The model under review builds one solid part; all positions refer to its coordinate system, in mm. Face numbers are marked on the shaded views. A direction names the side the tool comes from. Give positions to 0.01 mm unless a question says otherwise; leave off trailing zeros. Order: outer loops, then holes, each group sorted by start corner. A loop starts at its lowest first (then second) coordinate and runs counter-clockwise, first axis right, second up.
```python
from build123d import *

# Parameters (mm, degrees)
BOSS_EXTRUDE1_DEPTH     = 200
BOSS_EXTRUDE2_DEPTH     = 5
BOSS_EXTRUDE3_START     = 200
BOSS_EXTRUDE3_DEPTH     = 5
BOSS_EXTRUDE5_START     = -70
SKETCH12_W              = 5
SKETCH12_H              = 200
BOSS_EXTRUDE5_DEPTH     = 14
SKETCH13_R              = 1.75
SKETCH13_R_2            = 5
SKETCH13_W              = 98
SKETCH13_H              = 41
CUT_EXTRUDE7_DEPTH      = 1
CUT_EXTRUDE7_DEPTH_BACK = 85
SKETCH15_R              = 3
CUT_EXTRUDE8_DEPTH      = 3
SKETCH16_R              = 1.75
CUT_EXTRUDE9_DEPTH      = 111
CUT_EXTRUDE9_DEPTH_BACK = 111
CUT_EXTRUDE10_START     = -103
CUT_EXTRUDE10_DEPTH     = 3
CUT_EXTRUDE11_START     = 100
CUT_EXTRUDE11_DEPTH     = 3
SKETCH18_R              = 3
CUT_EXTRUDE12_DEPTH     = 3


with BuildPart() as part:
    # Sketch1 → Boss-Extrude1 (new body)
    with BuildSketch(Plane(origin=(0, 0, 0), x_dir=(1, 0, 0), z_dir=(0, 1, 0))):
        Polygon((0, 0), (100, 0), (110, 10), (110, 70), (100, 70), (100, 10), (0, 10), align=None)
    boss_extrude1 = extrude(amount=BOSS_EXTRUDE1_DEPTH)

    # Mirror1: Boss-Extrude1 across plane
    add(boss_extrude1.mirror(Plane(origin=(0, 0, 0), x_dir=(0, 0, 1), z_dir=(1, 0, 0))))

    # Sketch6 → Boss-Extrude2 (add)
    with BuildSketch(Plane(origin=(0, 0, 0), x_dir=(1, 0, 0), z_dir=(0, 1, 0))):
        Polygon((110, 70), (-110, 70), (-110, 10), (-100, 0), (100, 0), (110, 10), align=None)
    extrude(amount=-BOSS_EXTRUDE2_DEPTH)

    # Sketch6<2> → Boss-Extrude3 (add)
    with BuildSketch(Plane(origin=(0, 0, 0), x_dir=(1, 0, 0), z_dir=(0, 1, 0)).offset(BOSS_EXTRUDE3_START)):
        Polygon((110, 70), (-110, 70), (-110, 10), (-100, 0), (100, 0), (110, 10), align=None)
    extrude(amount=BOSS_EXTRUDE3_DEPTH)

    # Sketch12 → Boss-Extrude5 (add)
    with BuildSketch(Plane.XY.offset(BOSS_EXTRUDE5_START)):
        with Locations((102.5, 100)):
            Rectangle(SKETCH12_W, SKETCH12_H)
        with Locations((-102.5, 100)):
            Rectangle(SKETCH12_W, SKETCH12_H)
    extrude(amount=-BOSS_EXTRUDE5_DEPTH)

    # Sketch13 → Cut-Extrude7 (cut, two sides)
    with BuildSketch(Plane.XY) as cut_extrude7_sk:
        with Locations((-46.5, 165)):
            Circle(SKETCH13_R)
        with Locations((46.5, 165)):
            Circle(SKETCH13_R)
        with Locations((46.5, 110)):
            Circle(SKETCH13_R)
        with Locations((-46.5, 110)):
            Circle(SKETCH13_R)
        with Locations((32.75, 62.246184667)):
            Circle(SKETCH13_R)
        with Locations((-32.75, 62.246184667)):
            Circle(SKETCH13_R)
        with Locations((32.75, 21.746184667)):
            Circle(SKETCH13_R)
        with Locations((-32.75, 21.746184667)):
            Circle(SKETCH13_R)
        with Locations((24, 35.496184667)):
            Circle(SKETCH13_R_2)
        with Locations((-18.75, 35.496184667)):
            Circle(SKETCH13_R_2)
        with Locations((4.25, 35.496184667)):
            Circle(SKETCH13_R_2)
        with Locations((0, 137.5)):
            Rectangle(SKETCH13_W, SKETCH13_H)
    extrude(amount=CUT_EXTRUDE7_DEPTH, mode=Mode.SUBTRACT)
    extrude(cut_extrude7_sk.sketch, amount=-CUT_EXTRUDE7_DEPTH_BACK, mode=Mode.SUBTRACT)

    # Sketch15 → Cut-Extrude8 (cut)
    with BuildSketch(Plane.XY):
        with Locations((-46.5, 165)):
            Circle(SKETCH15_R)
        with Locations((46.5, 165)):
            Circle(SKETCH15_R)
        with Locations((46.5, 110)):
            Circle(SKETCH15_R)
        with Locations((-46.5, 110)):
            Circle(SKETCH15_R)
    extrude(amount=-CUT_EXTRUDE8_DEPTH, mode=Mode.SUBTRACT)

    # Sketch16 → Cut-Extrude9 (cut, two sides)
    with BuildSketch(Plane(origin=(0, 0, 0), x_dir=(0, 0, -1), z_dir=(1, 0, 0))) as cut_extrude9_sk:
        with Locations((79, 185)):
            Circle(SKETCH16_R)
        with Locations((79, 15)):
            Circle(SKETCH16_R)
    extrude(amount=CUT_EXTRUDE9_DEPTH, mode=Mode.SUBTRACT)
    extrude(cut_extrude9_sk.sketch, amount=-CUT_EXTRUDE9_DEPTH_BACK, mode=Mode.SUBTRACT)

    # Sketch17 → Cut-Extrude10 (cut)
    with BuildSketch(Plane(origin=(0, 0, 0), x_dir=(0, 0, -1), z_dir=(1, 0, 0)).offset(CUT_EXTRUDE10_START)):
        Polygon((75.535898385, 185), (77.267949192, 182), (80.732050808, 182), (82.464101615, 185), (80.732050808, 188), (77.267949192, 188), align=None)
        Polygon((75.690677898, 13.976092178), (78.232069134, 11.62208908), (81.541391236, 12.645996901), (82.309322102, 16.023907822), (79.767930866, 18.37791092), (76.458608764, 17.354003099), align=None)
    extrude(amount=CUT_EXTRUDE10_DEPTH, mode=Mode.SUBTRACT)

    # Sketch17<2> → Cut-Extrude11 (cut)
    with BuildSketch(Plane(origin=(0, 0, 0), x_dir=(0, 0, -1), z_dir=(1, 0, 0)).offset(CUT_EXTRUDE11_START)):
        Polygon((75.535898385, 185), (77.267949192, 182), (80.732050808, 182), (82.464101615, 185), (80.732050808, 188), (77.267949192, 188), align=None)
        Polygon((75.690677898, 13.976092178), (78.232069134, 11.62208908), (81.541391236, 12.645996901), (82.309322102, 16.023907822), (79.767930866, 18.37791092), (76.458608764, 17.354003099), align=None)
    extrude(amount=CUT_EXTRUDE11_DEPTH, mode=Mode.SUBTRACT)

    # Sketch18 → Cut-Extrude12 (cut)
    with BuildSketch(Plane.XY):
        with Locations((32.75, 62.246184667)):
            Circle(SKETCH18_R)
        with Locations((-32.75, 62.246184667)):
            Circle(SKETCH18_R)
        with Locations((-32.75, 21.746184667)):
            Circle(SKETCH18_R)
        with Locations((32.75, 21.746184667)):
            Circle(SKETCH18_R)
    extrude(amount=-CUT_EXTRUDE12_DEPTH, mode=Mode.SUBTRACT)


solid = part.part
```
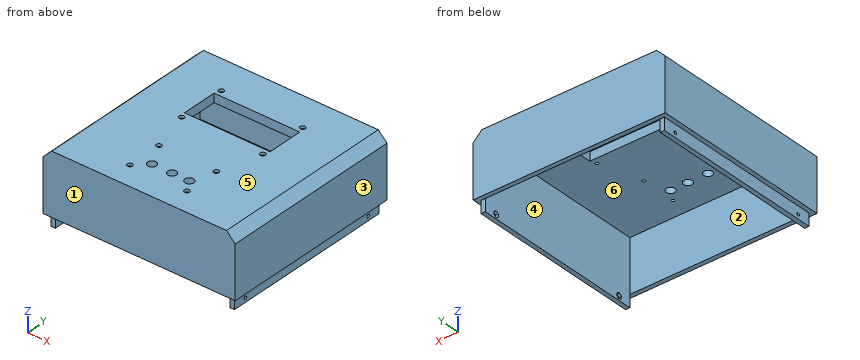
Item 1: Take a section at B-B (x = -18.75). Give the boundary of the cut face in (y, z).
Values found:
outline: (-5, -70) - (0, -70) - (0, -10) - (30.5, -10) - (30.5, 0) - (-5, 0) - close; (40.5, -10) - (117, -10) - (117, 0) - (40.5, 0) - close; (158, -10) - (200, -10) - (200, -70) - (205, -70) - (205, 0) - (158, 0) - close
Item 2: Take a section at D-D (x = 77.5). Give the boundary of the cut face in (y, z).
Values found:
outline: (-5, -70) - (0, -70) - (0, -10) - (200, -10) - (200, -70) - (205, -70) - (205, 0) - (-5, 0) - close
Item 3: Take a section at C-C (z = -54). Give the boundary of the cut face in (x, y).
Values found:
outline: (-110, -5) - (110, -5) - (110, 205) - (-110, 205) - close; hole (-100, 0) - (100, 0) - (100, 200) - (-100, 200) - close
Item 4: Take a section at A-A (y = 131). Give the boundary of the cut face in (x, z), and give its area (3 significant figures).
Values found:
outline: (-110, -70) - (-105, -70) - (-105, -84) - (-100, -84) - (-100, -10) - (-49, -10) - (-49, 0) - (-100, 0) - (-110, -10) - close; (49, -10) - (100, -10) - (100, -84) - (105, -84) - (105, -70) - (110, -70) - (110, -10) - (100, 0) - (49, 0) - close
area: 2,460 mm2
Item 5: For line 1 (Y direction, x = -104.6, z = -79); line 2 (Y direction, x = -90.5, z = -14); line 3 (X direction, y = 47.5, z = -18), list the stretches that pass through material, from the lowest coordinate up.
Values found:
line 1: y = 0 to 13.25, 16.75 to 183.25, 186.75 to 200
line 2: y = -5 to 0, 200 to 205
line 3: x = -110 to -100, 100 to 110
Item 6: For the marked faces 5 and 6, list the 3-axis set-ups (+Z, -Z, +X, -X, +Y, -Y) from which the entire face can be reached by the end or side of a thin tool; tool diameter is ignored.
Values found:
face 5: +Z, +X, -X, +Y, -Y
face 6: -Z
Item 7: Draft analysis for pull direction Y (two halves, no side actions). For the marked faces 1, 2, 3 and 4, state which applies: released by +Y, released by -Y, zero draft, split by the parting line, or undercut.
Values found:
face 1: released by -Y
face 2: undercut
face 3: zero draft
face 4: undercut
Item 8: Clearance check with flat-ended pins moving along their axes: pin 1 Ø12 at (x, y) = (-13, 78) entering from +Z; pin 2 Ø3.5 at (x, z) = (101, -79) entering from -Y; pin 3 Ø4 at (x, z) = (103.5, -75.5) entering from +Y; pin 4 Ø3 at (y, z) = (186, -78.5) entering from +X. State where each tip first meets the part, or that it passes through.
Values found:
pin 1: stops at z = 0
pin 2: stops at y = 0
pin 3: stops at y = 200
pin 4: stops at x = 105
